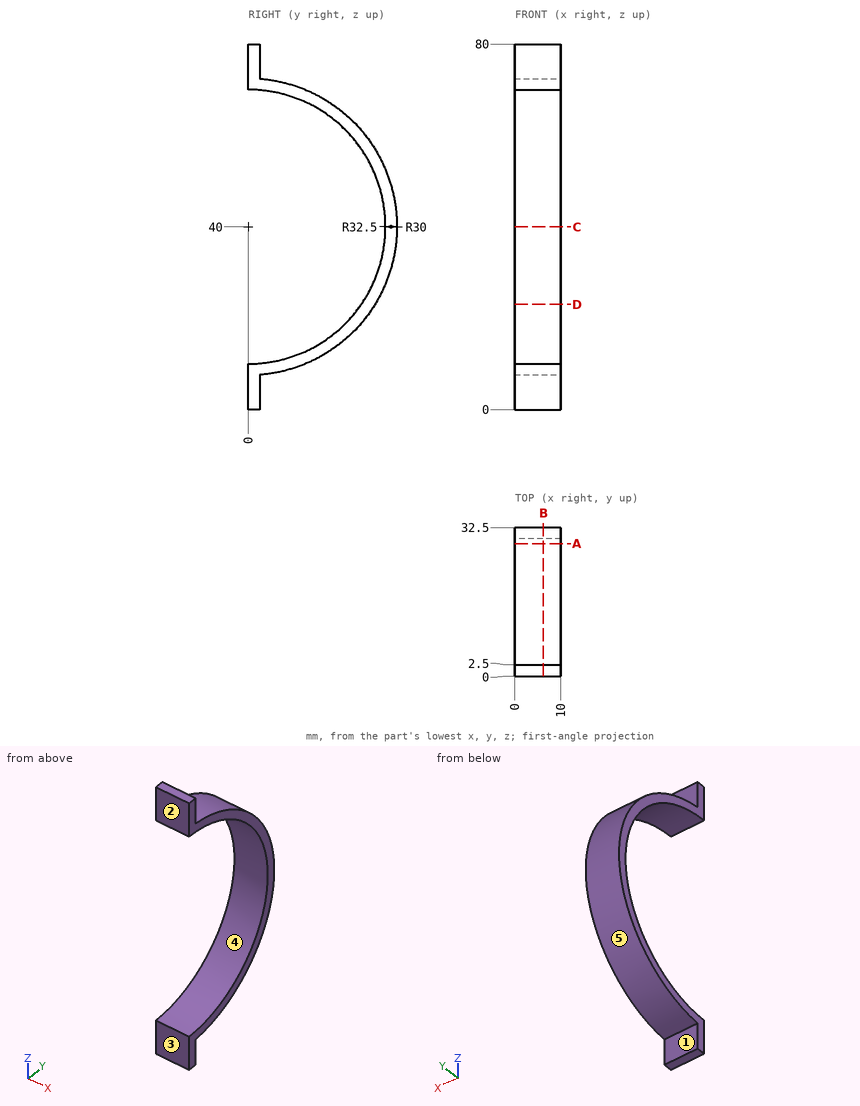
Geometry: see drawing. Coordinates: mm, zero at the bounding-box minimum. A direction names the side the tool comes from. Coordinates: 2 decimals unless noted, no trailing zeros. Loops run counter-clockwise (first coordinate to the right, second up) from the corner with the lowest first, then second, coordinate; pieces in that order, holes last.
(1) Section D-D on z = 23. Return the cut outline in (x, y).
(2) Section C-C on z = 40. Return the cut outline in (x, y).
(3) Section B-B on x = 6.25. Return the cut outline in (y, z), then the cut area to 3 significant figures.
(4) Set-up query: the marked faces 1 and 2. Return all of +Z, -Z, +X, -X, +Y, -Y with unobstructed straight access to the full face (end or side cutting, diameter ignored); none if empty.
(5) Material intervals for probe 1 along Y at (x, z) = (6.75, 76); probe 2 along Z at (x, y) = (5.5, 14); probe 3 along Z at (x, y) = (1.25, 10), sorted ascending.
(6) Section A-A on y = 29. Return the cut outline in (x, z), then the cut area to 3 significant figures.
(7) Pull-direction query (Z, two-part tool) for the marked faces 3, 4 and 5; classes: released by +Z, released by -Z, zero draft, split by the parting line, or undercut.
(8) First-contact query: pin 1 Ø4 at (x, y) = (8.5, 26) entering from +Z; pin 2 Ø5 at (x, z) = (7.5, 15) entering from -Y; pin 3 Ø5 at (x, y) = (5, 20) entering from -Z. Flat tips, straight axial feed; report the tip coordinate or a pass-through.
Data:
1. outline: (0, 24.72) - (10, 24.72) - (10, 27.7) - (0, 27.7) - close
2. outline: (0, 30) - (10, 30) - (10, 32.5) - (0, 32.5) - close
3. outline: (0, 0) - (2.5, 0) - (2.5, 7.6) arc R32.5 ccw to (2.5, 72.4) - (2.5, 80) - (0, 80) - (0, 70) arc R30 cw to (0, 10) - close
3. area: 283 mm2
4. face 1: -Z, +X, -X, +Y
4. face 2: +Z, -Z, +X, -X, -Y
5. probe 1: y = 0 to 2.5
5. probe 2: z = 10.67 to 13.47, 66.53 to 69.33
5. probe 3: z = 9.08 to 11.72, 68.28 to 70.92
6. outline: (0, 25.33) - (10, 25.33) - (10, 32.32) - (0, 32.32) - close; (0, 47.68) - (10, 47.68) - (10, 54.67) - (0, 54.67) - close
6. area: 140 mm2
7. face 3: zero draft
7. face 4: undercut
7. face 5: split by the parting line
8. pin 1: stops at z = 61.91
8. pin 2: stops at y = 11.99
8. pin 3: stops at z = 12.61
